Verification items for the finished model (mm, model axes). A direction names the side the tool comes from. Give positions to 0.01 mm unless a question says otherwise; leave off trailing zeros. Loops run counter-clockwise (first coordinate to the right, second up) from the corner with the lowest first, then second, coordinate; pieces in that order, holes last. Notation, with made-up numbers: (-36, -0.75) - (-19, -0.75) arc R10 cw to (-19, 15.25) - close; hole circle Ø6 at (13, -35). An arc over 180 degrees is marked (long way). Answer in a Markdown table with one row per item.
```python
from build123d import *

# Parameters (mm, degrees)
SKETCH1_R           = 6.25
BOSS_EXTRUDE1_DEPTH = 12
CUT_EXTRUDE1_REACH  = 14
SKETCH2_R           = 1.5
SKETCH3_R           = 4.1
CUT_EXTRUDE2_DEPTH  = 5.5
SKETCH4_R           = 4.1
CUT_EXTRUDE3_DEPTH  = 5.5
SKETCH5_W           = 0.25
SKETCH5_H           = 1
CUT_EXTRUDE4_DEPTH  = 0.4
BOSS_EXTRUDE2_DEPTH = 0.2
CHAMFER1_SIZE       = 0.4


with BuildPart() as part:
    # Sketch1 → Boss-Extrude1 (new body)
    with BuildSketch(Plane.XY):
        Circle(SKETCH1_R)
    extrude(amount=BOSS_EXTRUDE1_DEPTH)

    # Sketch2 → Cut-Extrude1 (cut, up to next)
    with BuildSketch(Plane.XY.offset(12), mode=Mode.PRIVATE) as cut_extrude1_sk1:
        Circle(SKETCH2_R)
    cut_extrude1_tool1 = extrude(cut_extrude1_sk1.sketch, amount=-CUT_EXTRUDE1_REACH, mode=Mode.PRIVATE) & part.part
    add(cut_extrude1_tool1.solids().sort_by_distance((0, 0, 12))[0], mode=Mode.SUBTRACT)

    # Sketch3 → Cut-Extrude2 (cut)
    with BuildSketch(Plane.XY.offset(12)):
        Circle(SKETCH3_R)
    extrude(amount=-CUT_EXTRUDE2_DEPTH, mode=Mode.SUBTRACT)

    # Sketch4 → Cut-Extrude3 (cut)
    with BuildSketch(Plane(origin=(0, 0, 0), x_dir=(-1, 0, 0), z_dir=(0, 0, -1))):
        Circle(SKETCH4_R)
    extrude(amount=-CUT_EXTRUDE3_DEPTH, mode=Mode.SUBTRACT)

    # Sketch5 → Cut-Revolve1 (revolve, cut)
    with BuildSketch(Plane(origin=(0, 0, 0), x_dir=(1, 0, 0), z_dir=(0, 1, 0))):
        with Locations((4.225, -2.9)):
            Rectangle(SKETCH5_W, SKETCH5_H)
        with Locations((4.225, -9.1)):
            Rectangle(SKETCH5_W, SKETCH5_H)
    revolve(axis=Axis((0, 0, 12), (0, 0, -1)), mode=Mode.SUBTRACT)

    # Sketch6 → Cut-Extrude4 (cut)
    with BuildSketch(Plane(origin=(0, 0, 5.5), x_dir=(-1, 0, 0), z_dir=(0, 0, -1))):
        with BuildLine():
            ThreePointArc((-3.815756806, 1.5), (-4.1, 0), (-3.815756806, -1.5))
            Line((-3.815756806, -1.5), (0, -1.5))
            ThreePointArc((0, -1.5), (-1.5, 0), (0, 1.5))
            Line((0, 1.5), (-3.815756806, 1.5))
        make_face()
        with BuildLine():
            ThreePointArc((1.5, 0), (1.060660172, -1.060660172), (0, -1.5))
            Line((0, -1.5), (3.815756806, -1.5))
            ThreePointArc((3.815756806, -1.5), (4.028312482, -0.763346938), (4.1, 0))
            ThreePointArc((4.1, 0), (4.028312482, 0.763346938), (3.815756806, 1.5))
            Line((3.815756806, 1.5), (0, 1.5))
            ThreePointArc((0, 1.5), (1.060660172, 1.060660172), (1.5, 0))
        make_face()
    extrude(amount=-CUT_EXTRUDE4_DEPTH, mode=Mode.SUBTRACT)

    # Sketch7 → Boss-Extrude2 (add)
    with BuildSketch(Plane(origin=(0, 0, 5.9), x_dir=(-1, 0, 0), z_dir=(0, 0, -1))):
        with BuildLine():
            Line((-1.5, 0), (-1.5, 1.5))
            Line((-1.5, 1.5), (-3.815756806, 1.5))
            ThreePointArc((-3.815756806, 1.5), (-4.1, 0), (-3.815756806, -1.5))
            Line((-3.815756806, -1.5), (-1.5, -1.5))
            Line((-1.5, -1.5), (-1.5, 0))
        make_face()
        with BuildLine():
            ThreePointArc((3.815756806, -1.5), (4.1, 0), (3.815756806, 1.5))
            Line((3.815756806, 1.5), (1.5, 1.5))
            Line((1.5, 1.5), (1.5, 0))
            Line((1.5, 0), (1.5, -1.5))
            Line((1.5, -1.5), (3.815756806, -1.5))
        make_face()
    extrude(amount=BOSS_EXTRUDE2_DEPTH)

    # Chamfer1
    chamfer1_edges = [part.edges().sort_by_distance(p)[0] for p in [
        (-4.1, 0, 12),
        (4.1, 0, 0),
        (-6.25, 0, 0),
        (-6.25, 0, 12),
    ]]
    chamfer(chamfer1_edges, length=CHAMFER1_SIZE)


solid = part.part
```
Q1. Sectioned sample at B-B (z = 3). Record the cut outline in (x, y).
Completed:
| item | result |
|---|---|
| outline | circle Ø12.5 at (0, 0); hole circle Ø8.7 at (0, 0) |
Q2. Sectioned sample at A-A (z = 7.75). Record the cut outline in (x, y), and give its area (3 significant figures).
Completed:
| item | result |
|---|---|
| outline | circle Ø12.5 at (0, 0); hole circle Ø8.2 at (0, 0) |
| area | 69.9 mm^2 |
Q3. Go/stop test with flat-tipped pins: P1, Ø1.5, axis at y = 3, z = 1.5, coming from the +X side; P2, Ø6, axis at y = -2.5, z = 7, coming from the +X side; P3, Ø0.8, axis at x = 2.5, y = -0.5, coming from the -Z side; P4, Ø1, axis at y = -4, z = 6, coming from the -X side. Record where each tip stops, or that it passes through.
Completed:
| item | result |
|---|---|
| P1 | x = 5.83 |
| P2 | x = 6.25 |
| P3 | z = 5.7 |
| P4 | x = -5.18 |
Q4. Tool access check on faces 1 (the face through (5.96, 1.88, 5.92)), 2 (the face through (-3, 0, 5.7)), 3 (the face through (2, 0, 6.5)). Record the directions out of +Z, -Z, +X, -X, +Y, -Y that give a thin tool (end or side, any length) a straight path to the whole face; none if there is none.
Completed:
| item | result |
|---|---|
| face 1 | +Z, -Z |
| face 2 | -Z |
| face 3 | +Z |
Q5. Thickness scan on line 1 (Y direction, x = 0, z = 1.8); line 2 (Z direction, x = -3, y = 3); line 3 (Y direction, x = 0, z = 3.05). Record the ranges inside material, lowest first.
Completed:
| item | result |
|---|---|
| line 1 | -6.25 to -4.1, 4.1 to 6.25 |
| line 2 | 0.26 to 2.4, 3.4 to 8.6, 9.6 to 11.74 |
| line 3 | -6.25 to -4.35, 4.35 to 6.25 |
